Read the model definition and answer for the solid it produces. Units are mm, in the model's axes. Face numbers are marked on the shaded views. A direction names the side the tool comes from. Give positions to 0.01 mm unless a question says otherwise; leave off trailing zeros. Order: outer loops, then holes, each group sorted by start corner. A loop starts at its lowest first (then second) coordinate and runs counter-clockwise, first axis right, second up.
Item 1: A cutting plane is placed at A-A (y = 0). Write down the section's boundary in (x, z), plus the area to 3 significant figures.
Item 2: A cutting plane is placed at C-C (x = 3.75). Write down the section's boundary in (y, z), plus the area to 3 significant figures.
Item 3: Given pin 1 Ø3 at (x, z) = (0, 18.5) entering from +Y; pin 2 Ø1.5 at (x, z) = (-1.5, 18.5) entering from -Y; pin 3 Ø2 at (x, z) = (1.5, 23.5) entering from -Y, each flat-ended and moving along its own axis, determine where each tip first touches the part or whether it passes through.
Item 4: The mould has two halves that part along Z. Classify the marked faces 1, 2, 3 and 4: +Z half, -Z half, draft (parallel to the pull), parting line (faces both ways), or undercut.
Item 5: Which of the six approach directions +Z, -Z, +X, -X, +Y, -Y give full straight-line access (tool end or side, diameter ignored) to the marked faces 5, 6, 7, 8 and 9?
Item 6: A cutting plane is placed at D-D (z = 16.25). Write down the section's boundary in (x, y).
Item 7: A cutting plane is placed at B-B (z = 25.75). Write down the section's boundary in (x, y) (3 decimals), plus the area to 3 significant figures.
Item 8: Find the intervals of material crossed by line 1 along Z through (x, y) = (-2.75, -2.5); line 2 along Z through (x, y) = (-1, 3); line 3 along Z through (x, y) = (-2.5, -2.5), in increasing order.
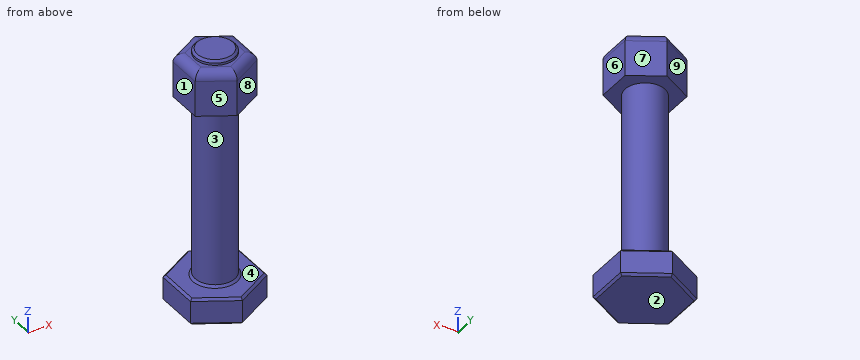
from build123d import *

# Parameters (mm, degrees)
PAD_DEPTH    = 3
SKETCH001_R  = 2.25
PAD001_DEPTH = 26
PAD002_START = -0.5
PAD002_DEPTH = 5
FILLET_R     = 1
CHAMFER_SIZE = 0.25


with BuildPart() as part:
    # Sketch → Pad (new body)
    with BuildSketch(Plane.XY):
        Polygon((0, 5), (-4.330127, 2.5), (-4.330127, -2.5), (0, -5), (4.330127, -2.5), (4.330127, 2.5), align=None)
    extrude(amount=PAD_DEPTH)

    # Sketch001 (on Face8 of Pad) → Pad001 (join)
    with BuildSketch(Plane.XY.offset(3)):
        Circle(SKETCH001_R)
    extrude(amount=PAD001_DEPTH)

    # Sketch002 (on Face10 of Pad001) → Pad002 (join)
    with BuildSketch(Plane.XY.offset(29).offset(PAD002_START)):
        Polygon((0, 4.03), (-3.490082, 2.015), (-3.490082, -2.015), (0, -4.03), (3.490082, -2.015), (3.490082, 2.015), align=None)
    extrude(amount=-PAD002_DEPTH)

    # Fillet
    fillet_edges = [part.edges().sort_by_distance(p)[0] for p in [
        (1.745041, -3.0225, 28.5),
        (3.490082, 0, 28.5),
        (1.745041, 3.0225, 28.5),
        (-1.745041, 3.0225, 28.5),
        (-3.490082, 0, 28.5),
        (-1.745041, -3.0225, 28.5),
    ]]
    fillet(fillet_edges, radius=FILLET_R)

    # Chamfer
    chamfer_edges = [part.edges().sort_by_distance(p)[0] for p in [
        (-2.165064, 3.75, 0),
        (-4.330127, 0, 0),
        (-2.165064, -3.75, 0),
        (2.165064, -3.75, 0),
        (4.330127, 0, 0),
        (2.165064, 3.75, 0),
        (-2.165064, 3.75, 3),
        (2.165064, 3.75, 3),
        (-4.330127, 0, 3),
        (4.330127, 0, 3),
        (-2.165064, -3.75, 3),
        (2.165064, -3.75, 3),
        (-2.25, 0, 3),
        (-2.25, 0, 29),
    ]]
    chamfer(chamfer_edges, length=CHAMFER_SIZE)


solid = part.part
Response values:
1. outline: (-4.33, 0.25) - (-4.08, 0) - (4.08, 0) - (4.33, 0.25) - (4.33, 2.75) - (4.08, 3) - (2.5, 3) - (2.25, 3.25) - (2.25, 23.5) - (3.49, 23.5) - (3.49, 27.5) arc R1 ccw to (2.49, 28.5) - (2.25, 28.5) - (2.25, 28.75) - (2, 29) - (-2, 29) - (-2.25, 28.75) - (-2.25, 28.5) - (-2.49, 28.5) arc R1 ccw to (-3.49, 27.5) - (-3.49, 23.5) - (-2.25, 23.5) - (-2.25, 3.25) - (-2.5, 3) - (-4.08, 3) - (-4.33, 2.75) - close
1. area: 155 mm2
2. outline: (-2.83, 0.25) - (-2.55, 0) - (2.55, 0) - (2.83, 0.25) - (2.83, 2.75) - (2.55, 3) - (-2.55, 3) - (-2.83, 2.75) - close
2. area: 16.9 mm2
3. pin 1: stops at y = 2.25
3. pin 2: stops at y = -2.12
3. pin 3: stops at y = -3.74
4. face 1: draft
4. face 2: -Z half
4. face 3: undercut
4. face 4: undercut
5. face 5: +Z, -X, -Y
5. face 6: +Z, +X, +Y, -Y
5. face 7: +Z, +X, +Y
5. face 8: +Z, +X, -Y
5. face 9: +Z, -X, +Y
6. outline: circle Ø4.5 at (0, 0)
7. outline: (-3.49, -2.015) - (0, -4.03) - (3.49, -2.015) - (3.49, 2.015) - (0, 4.03) - (-3.49, 2.015) - close
7. area: 42.2 mm2
8. line 1: z = 0 to 3
8. line 2: z = 0 to 3, 23.5 to 28.29
8. line 3: z = 0 to 3, 23.5 to 27.88
